Build history of the part. All positions in model axes, mm. Coordinates: 2 decimals unless noted, no trailing zeros. Write each loop counter-clockwise with the first axis right and the second up, starting at its lowest first coordinate (ties: lowest second). Pieces come first, ordered by that corner, then holes.
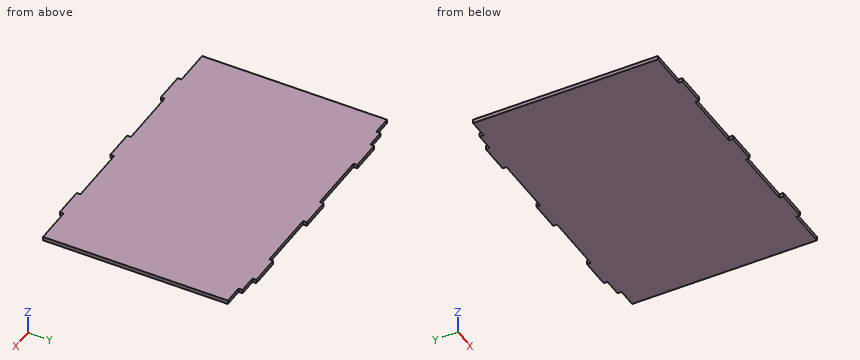
Autodesk Inventor part; units mm, degrees
ref_plane "YZ Plane" through (0, 0, 0) normal (1, 0, 0) x (0, 1, 0)
ref_plane "XZ Plane" through (0, 0, 0) normal (0, 1, 0) x (-1, 0, 0)
ref_plane "XY Plane" through (0, 0, 0) normal (0, 0, 1) x (1, 0, 0)
sketch "Sketch1" plane through (0, 0, 0) normal (0, 0, 1) x (1, 0, 0)
  line L0 (-38.1107, 23.9821) -> (441.9493, 23.9821)
  line L1 (441.9493, 23.9821) -> (441.9493, -289.7079)
  line L2 (441.9493, -289.7079) -> (-38.1107, -289.7079)
  line L3 (-38.1107, -289.7079) -> (-38.1107, 23.9821)
  line L4 (-38.1107, -289.7079) -> (227.3193, -289.7079)
  line L5 (227.3193, -289.7079) -> (176.5193, -289.7079)
  line L6 (176.5193, -289.7079) -> (176.5193, -296.0579)
  line L7 (176.5193, -296.0579) -> (227.3193, -296.0579)
  line L8 (227.3193, -296.0579) -> (227.3193, -289.7079)
  line L9 (227.3193, -289.7079) -> (328.9193, -289.7079)
  line L10 (328.9193, -289.7079) -> (74.9193, -289.7079)
  line L11 (74.9193, -289.7079) -> (24.1193, -289.7079)
  line L12 (24.1193, -289.7079) -> (24.1193, -296.0579)
  line L13 (24.1193, -296.0579) -> (74.9193, -296.0579)
  line L14 (74.9193, -296.0579) -> (74.9193, -289.7079)
  line L15 (328.9193, -289.7079) -> (379.7193, -289.7079)
  line L16 (379.7193, -289.7079) -> (379.7193, -296.0579)
  line L17 (379.7193, -296.0579) -> (328.9193, -296.0579)
  line L18 (328.9193, -296.0579) -> (328.9193, -289.7079)
  line L19 (24.1193, 23.9821) -> (74.9193, 23.9821)
  line L20 (74.9193, 23.9821) -> (74.9193, 30.3321)
  line L21 (74.9193, 30.3321) -> (24.1193, 30.3321)
  line L22 (24.1193, 30.3321) -> (24.1193, 23.9821)
  line L23 (176.5193, 23.9821) -> (227.3193, 23.9821)
  line L24 (227.3193, 23.9821) -> (227.3193, 30.3321)
  line L25 (227.3193, 30.3321) -> (176.5193, 30.3321)
  line L26 (176.5193, 30.3321) -> (176.5193, 23.9821)
  line L27 (328.9193, 23.9821) -> (379.7193, 23.9821)
  line L28 (379.7193, 23.9821) -> (379.7193, 30.3321)
  line L29 (379.7193, 30.3321) -> (328.9193, 30.3321)
  line L30 (328.9193, 30.3321) -> (328.9193, 23.9821)
  line L31 (-38.1107, 23.9821) -> (-6.1067, 23.9821)
  line L32 (-6.1067, 23.9821) -> (-6.1067, 17.3781)
  line L33 (-6.1067, 17.3781) -> (-38.1107, 17.3781)
  line L34 (-38.1107, 17.3781) -> (-38.1107, 23.9821)
  line L35 (441.9493, 23.9821) -> (409.9453, 23.9821)
  line L36 (409.9453, 23.9821) -> (409.9453, 17.3781)
  line L37 (409.9453, 17.3781) -> (441.9493, 17.3781)
  line L38 (441.9493, 17.3781) -> (441.9493, 23.9821)
  point P0 (0, 0)
  dimension "d0" = 480.06
  dimension "d1" = 313.69
  dimension "d2" = 265.43
  dimension "d3" = 50.8
  dimension "d4" = 6.35
  dimension "d5" = 101.6
  dimension "d6" = 254
  dimension "d7" = 50.8
  dimension "d8" = 50.8
  dimension "d9" = 6.35
  dimension "d10" = 32.004
  dimension "d11" = 6.604
  dimension "d12" = 32.004
extrude "Extrusion1" add sketch "Sketch1" along normal blind 6.35 contours L0 L36 L37 L1 L2 L3 L33 L32 | L22 L21 L20 L0 | L2 L14 L13 L12 | L26 L25 L24 L0 | L2 L8 L7 L6 | L30 L29 L28 L0 | L2 L16 L17 L18
properties part number "it shelf"
1. Flat gauge pins, fed straight in: pin 1 (3 mm diameter, centred on y = 27.5, z = 4.5, fed in from +X); pin 2 (3 mm diameter, centred on x = 397.5, z = 3, fed in from +Y); pin 3 (1.9 mm diameter, centred on y = 28.5, z = 3, fed in from -X). Where does each tip first touch, or does it go through?
Computed values:
pin 1: stops at x = 379.72
pin 2: stops at y = 23.98
pin 3: stops at x = 24.12
2. Probe line 1 along Y through (x, z) = (105, 6). List the from-to ranges inside material, lowest first.
Computed values:
line 1: y = -289.71 to 23.98
3. Saw through at B-B on x = 168. List the corners of the cut face in (y, z).
Computed values:
outline: (-289.71, 0) - (23.98, 0) - (23.98, 6.35) - (-289.71, 6.35) - close
